```python
from build123d import *

# Parameters (mm, degrees)
SKETCH1_R           = 25
SKETCH1_R_2         = 1.25
SKETCH1_R_3         = 7.5
BOSS_EXTRUDE1_DEPTH = 5
BOSS_EXTRUDE2_DEPTH = 20
BOSS_EXTRUDE3_DEPTH = 30
SKETCH4_R           = 1.25
SKETCH4_R_2         = 20
BOSS_EXTRUDE4_DEPTH = 5
BOSS_EXTRUDE5_DEPTH = 8


with BuildPart() as part:
    # Sketch1 → Boss-Extrude1 (new body)
    with BuildSketch(Plane.XY):
        Circle(SKETCH1_R)
        with Locations((-12.85, 0)):
            Circle(SKETCH1_R_2, mode=Mode.SUBTRACT)
        with Locations((-6.425, 11.128426439)):
            Circle(SKETCH1_R_2, mode=Mode.SUBTRACT)
        with Locations((6.425, 11.128426439)):
            Circle(SKETCH1_R_2, mode=Mode.SUBTRACT)
        with Locations((12.85, 0)):
            Circle(SKETCH1_R_2, mode=Mode.SUBTRACT)
        with Locations((6.425, -11.128426439)):
            Circle(SKETCH1_R_2, mode=Mode.SUBTRACT)
        with Locations((-6.425, -11.128426439)):
            Circle(SKETCH1_R_2, mode=Mode.SUBTRACT)
        Circle(SKETCH1_R_3, mode=Mode.SUBTRACT)
    extrude(amount=BOSS_EXTRUDE1_DEPTH)

    # Sketch2 → Boss-Extrude2 (add)
    with BuildSketch(Plane(origin=(0, 0, 0), x_dir=(-1, 0, 0), z_dir=(0, 0, -1))):
        with BuildLine():
            Line((-15.244012286, 6.314276634), (-23.096988313, 9.567085809))
            ThreePointArc((-23.096988313, 9.567085809), (-25, 0), (-23.096988313, -9.567085809))
            Line((-23.096988313, -9.567085809), (-15.244012286, -6.314276634))
            ThreePointArc((-15.244012286, -6.314276634), (-16.5, 0), (-15.244012286, 6.314276634))
        make_face()
        with BuildLine():
            Line((6.314276634, 15.244012286), (9.567085809, 23.096988313))
            ThreePointArc((9.567085809, 23.096988313), (0, 25), (-9.567085809, 23.096988313))
            Line((-9.567085809, 23.096988313), (-6.314276634, 15.244012286))
            ThreePointArc((-6.314276634, 15.244012286), (0, 16.5), (6.314276634, 15.244012286))
        make_face()
        with BuildLine():
            ThreePointArc((25, 0), (24.51963201, 4.87725805), (23.096988313, 9.567085809))
            Line((23.096988313, 9.567085809), (15.244012286, 6.314276634))
            ThreePointArc((15.244012286, 6.314276634), (16.5, 0), (15.244012286, -6.314276634))
            Line((15.244012286, -6.314276634), (23.096988313, -9.567085809))
            ThreePointArc((23.096988313, -9.567085809), (24.51963201, -4.87725805), (25, 0))
        make_face()
        with BuildLine():
            ThreePointArc((-9.567085809, -23.096988313), (0, -25), (9.567085809, -23.096988313))
            Line((9.567085809, -23.096988313), (6.314276634, -15.244012286))
            ThreePointArc((6.314276634, -15.244012286), (0, -16.5), (-6.314276634, -15.244012286))
            Line((-6.314276634, -15.244012286), (-9.567085809, -23.096988313))
        make_face()
    extrude(amount=BOSS_EXTRUDE2_DEPTH)

    # Sketch3 → Boss-Extrude3 (add)
    with BuildSketch(Plane.XY.offset(5)):
        with BuildLine():
            Line((7.653668647, 18.47759065), (9.567085809, 23.096988313))
            ThreePointArc((9.567085809, 23.096988313), (0, 25), (-9.567085809, 23.096988313))
            Line((-9.567085809, 23.096988313), (-7.653668647, 18.47759065))
            ThreePointArc((-7.653668647, 18.47759065), (0, 20), (7.653668647, 18.47759065))
        make_face()
        with BuildLine():
            ThreePointArc((25, 0), (24.51963201, 4.87725805), (23.096988313, 9.567085809))
            Line((23.096988313, 9.567085809), (18.47759065, 7.653668647))
            ThreePointArc((18.47759065, 7.653668647), (20, 0), (18.47759065, -7.653668647))
            Line((18.47759065, -7.653668647), (23.096988313, -9.567085809))
            ThreePointArc((23.096988313, -9.567085809), (24.51963201, -4.87725805), (25, 0))
        make_face()
        with BuildLine():
            Line((-7.653668647, -18.47759065), (-9.567085809, -23.096988313))
            ThreePointArc((-9.567085809, -23.096988313), (0, -25), (9.567085809, -23.096988313))
            Line((9.567085809, -23.096988313), (7.653668647, -18.47759065))
            ThreePointArc((7.653668647, -18.47759065), (0, -20), (-7.653668647, -18.47759065))
        make_face()
        with BuildLine():
            Line((-18.47759065, 7.653668647), (-23.096988313, 9.567085809))
            ThreePointArc((-23.096988313, 9.567085809), (-25, 0), (-23.096988313, -9.567085809))
            Line((-23.096988313, -9.567085809), (-18.47759065, -7.653668647))
            ThreePointArc((-18.47759065, -7.653668647), (-20, 0), (-18.47759065, 7.653668647))
        make_face()
    extrude(amount=BOSS_EXTRUDE3_DEPTH)

    # Sketch4 → Boss-Extrude4 (add)
    with BuildSketch(Plane.XY.offset(35)):
        with BuildLine():
            ThreePointArc((22.507298661, 18.971764755), (21.760152434, 21.760152434), (18.971764755, 22.507298661))
            ThreePointArc((18.971764755, 22.507298661), (0, 29.436479935), (-18.971764755, 22.507298661))
            ThreePointArc((-18.971764755, 22.507298661), (-21.760152434, 21.760152434), (-22.507298661, 18.971764755))
            ThreePointArc((-22.507298661, 18.971764755), (-29.436479935, 0), (-22.507298661, -18.971764755))
            ThreePointArc((-22.507298661, -18.971764755), (-21.760152434, -21.760152434), (-18.971764755, -22.507298661))
            ThreePointArc((-18.971764755, -22.507298661), (0, -29.436479935), (18.971764755, -22.507298661))
            ThreePointArc((18.971764755, -22.507298661), (21.760152434, -21.760152434), (22.507298661, -18.971764755))
            ThreePointArc((22.507298661, -18.971764755), (29.436479935, 0), (22.507298661, 18.971764755))
        make_face()
        with Locations((-19.718910982, -19.718910982)):
            Circle(SKETCH4_R, mode=Mode.SUBTRACT)
        with Locations((19.718910982, -19.718910982)):
            Circle(SKETCH4_R, mode=Mode.SUBTRACT)
        with Locations((-19.718910982, 19.718910982)):
            Circle(SKETCH4_R, mode=Mode.SUBTRACT)
        Circle(SKETCH4_R_2, mode=Mode.SUBTRACT)
        with Locations((19.718910982, 19.718910982)):
            Circle(SKETCH4_R, mode=Mode.SUBTRACT)
    extrude(amount=BOSS_EXTRUDE4_DEPTH)

    # Sketch5 → Boss-Extrude5 (add)
    with BuildSketch(Plane.XY.offset(40)):
        with BuildLine():
            ThreePointArc((11.264853178, 27.195761321), (0, 29.436479935), (-11.264853178, 27.195761321))
            Line((-11.264853178, 27.195761321), (-8.801718944, 21.249229248))
            ThreePointArc((-8.801718944, 21.249229248), (0, 23), (8.801718944, 21.249229248))
            Line((8.801718944, 21.249229248), (11.264853178, 27.195761321))
        make_face()
        with BuildLine():
            Line((21.249229248, -8.801718944), (27.195761321, -11.264853178))
            ThreePointArc((27.195761321, -11.264853178), (29.436479935, 0), (27.195761321, 11.264853178))
            Line((27.195761321, 11.264853178), (21.249229248, 8.801718944))
            ThreePointArc((21.249229248, 8.801718944), (23, 0), (21.249229248, -8.801718944))
        make_face()
        with BuildLine():
            Line((-8.801718944, -21.249229248), (-11.264853178, -27.195761321))
            ThreePointArc((-11.264853178, -27.195761321), (0, -29.436479935), (11.264853178, -27.195761321))
            Line((11.264853178, -27.195761321), (8.801718944, -21.249229248))
            ThreePointArc((8.801718944, -21.249229248), (0, -23), (-8.801718944, -21.249229248))
        make_face()
        with BuildLine():
            Line((-21.249229248, 8.801718944), (-27.195761321, 11.264853178))
            ThreePointArc((-27.195761321, 11.264853178), (-29.436479935, 0), (-27.195761321, -11.264853178))
            Line((-27.195761321, -11.264853178), (-21.249229248, -8.801718944))
            ThreePointArc((-21.249229248, -8.801718944), (-23, 0), (-21.249229248, 8.801718944))
        make_face()
    extrude(amount=BOSS_EXTRUDE5_DEPTH)


solid = part.part
```
Build history of the part. All positions in model axes, mm. A direction names the side the tool comes from. Round coordinates to 2 decimals unless told otherwise and drop trailing zeros. Order: outer loops, then holes, each group sorted by start corner. A loop starts at its lowest first (then second) coordinate and runs counter-clockwise, first axis right, second up. Notation, with made-up numbers: (9.25, 45.5) -> (27.25, 45.5) arc R18 cw to (27.25, 55.5) -> close; hole circle Ø1 at (35.5, -20.75). An arc over 180 degrees is marked (long way). Answer in a Markdown table with one row per item.
1) Wall check: L1, parallel to Y at x = 0, z = -4.5; L2, parallel to Y at x = 0, z = 28; L3, parallel to Z at x = 11, y = 20.5. Give the ranges that are in metal, low to high.
Values:
| item | result |
|---|---|
| L1 | -25 to -16.5, 16.5 to 25 |
| L2 | -25 to -20, 20 to 25 |
| L3 | 0 to 5, 35 to 40 |
2) Which spindle directions (+Z, -Z, +X, -X, +Y, -Y) get a long thin tool onto all of the face, cutting with end or side? Do faces 4 (the cylindrical face through (23, 0, 44)), 5 (the flat face through (24.181, -10.016, 43.944)), 6 (the flat face through (-24.181, 10.016, 43.944)), 7 (the flat face through (-5.5, 5.5, 5)), 8 (the cylindrical face through (-16.5, 0.1, -9.9)). Say none if no direction does.
Values:
| item | result |
|---|---|
| face 4 | +Z |
| face 5 | +Z, -Y |
| face 6 | +Z, +Y |
| face 7 | none |
| face 8 | -Z |
3) Mould opens along X. For faces 1 (the flat face through (8.624, -20.82, 19.79)), 2 (the flat face through (0, 20, -20)), 3 (the flat face through (20.82, 8.624, 19.79)) say: released by +X, released by -X, zero draft, split by the parting line, or undercut.
Values:
| item | result |
|---|---|
| face 1 | released by +X |
| face 2 | zero draft |
| face 3 | undercut |
4) Band-saw the part on D-D on z = -10. Give the cut face in (x, y).
Values:
| item | result |
|---|---|
| outline | (-23.1, -9.57) -> (-15.24, -6.31) arc R16.5 cw to (-15.24, 6.31) -> (-23.1, 9.57) arc R25 ccw to start; (-9.57, -23.1) arc R25 ccw to (9.57, -23.1) -> (6.31, -15.24) arc R16.5 cw to (-6.31, -15.24) -> close; (-9.57, 23.1) -> (-6.31, 15.24) arc R16.5 cw to (6.31, 15.24) -> (9.57, 23.1) arc R25 ccw to start; (15.24, -6.31) -> (23.1, -9.57) arc R25 ccw to (23.1, 9.57) -> (15.24, 6.31) arc R16.5 cw to start |
5) Band-saw the part on B-B on z = 7. Give the cut face in (x, y), and give its area (3 significant figures).
Values:
| item | result |
|---|---|
| outline | (-23.1, -9.57) -> (-18.48, -7.65) arc R20 cw to (-18.48, 7.65) -> (-23.1, 9.57) arc R25 ccw to start; (-9.57, -23.1) arc R25 ccw to (9.57, -23.1) -> (7.65, -18.48) arc R20 cw to (-7.65, -18.48) -> close; (-9.57, 23.1) -> (-7.65, 18.48) arc R20 cw to (7.65, 18.48) -> (9.57, 23.1) arc R25 ccw to start; (18.48, -7.65) -> (23.1, -9.57) arc R25 ccw to (23.1, 9.57) -> (18.48, 7.65) arc R20 cw to start |
| area | 353 mm2 |
6) Pin check, flat tips, straight feed: P1, Ø6, axis at y = -1.5, z = 13, coming from the +X side; P2, Ø4, axis at x = -19.72, y = -19.72, coming from the -Z side; P3, Ø2, axis at x = -19, z = 11.5, coming from the +Y side. Stop position of each tip, or through.
Values:
| item | result |
|---|---|
| P1 | x = 25 |
| P2 | z = 35 |
| P3 | y = 8.28 |
7) Band-saw the part on A-A on x = 0. Give the cut face in (y, z).
Values:
| item | result |
|---|---|
| outline | (-29.44, 35) -> (-25, 35) -> (-25, -20) -> (-16.5, -20) -> (-16.5, 0) -> (-7.5, 0) -> (-7.5, 5) -> (-20, 5) -> (-20, 40) -> (-23, 40) -> (-23, 48) -> (-29.44, 48) -> close; (7.5, 0) -> (16.5, 0) -> (16.5, -20) -> (25, -20) -> (25, 35) -> (29.44, 35) -> (29.44, 48) -> (23, 48) -> (23, 40) -> (20, 40) -> (20, 5) -> (7.5, 5) -> close |
8) Band-saw the part on C-C on y = -2.5. Give the cut face in (x, z).
Values:
| item | result |
|---|---|
| outline | (-29.33, 35) -> (-24.87, 35) -> (-24.87, -20) -> (-16.31, -20) -> (-16.31, 0) -> (-7.07, 0) -> (-7.07, 5) -> (-19.84, 5) -> (-19.84, 40) -> (-22.86, 40) -> (-22.86, 48) -> (-29.33, 48) -> close; (7.07, 0) -> (16.31, 0) -> (16.31, -20) -> (24.87, -20) -> (24.87, 35) -> (29.33, 35) -> (29.33, 48) -> (22.86, 48) -> (22.86, 40) -> (19.84, 40) -> (19.84, 5) -> (7.07, 5) -> close |
